Input: part model. Units: mm. Frame: model coordinates. A direction names the side the tool comes from. Coordinates: 2 decimals unless noted, no trailing zeros. Write each loop counter-clockwise with the first axis right and the second up, starting at its lowest first coordinate (ties: lowest second). Pieces come first, ordered by that corner, then holes. Notation, with made-up numbers: M -40,70.5 L -11,70.5 A25 cw -11,99.5 Z; hole C -30,-18.75 d6. An arc over 180 degrees is marked long. Answer as a JSON object with one key per item and string values. Group by question number.
from build123d import *

# Parameters (mm, degrees)
F0_W      = 20
F0_H      = 20
F0_R      = 3.5
F1_DEPTH  = 20
F2_R      = 3.5
F3_DEPTH  = 20
F4_R      = 3.5
F5_DEPTH  = 20
F6_R      = 5.5
F6_R_2    = 3.5
F7_DEPTH  = 16.5
F8_R      = 5.5
F9_DEPTH  = 16.5
F10_R     = 5.5
F11_DEPTH = 16.5


with BuildPart() as f1:
    # F0 (on Top) → F1 (new body)
    with BuildSketch(Plane.XY):
        Rectangle(F0_W, F0_H)
        Circle(F0_R, mode=Mode.SUBTRACT)
    extrude(amount=F1_DEPTH)

    # F2 (on face) → F3 (cut)
    with BuildSketch(Plane.XZ.offset(10)):
        with Locations((0, 10)):
            Circle(F2_R)
    extrude(amount=-F3_DEPTH, mode=Mode.SUBTRACT)

    # F4 (on face) → F5 (cut)
    with BuildSketch(Plane(origin=(-10, 0, 0), x_dir=(0, -1, 0), z_dir=(-1, 0, 0))):
        with Locations((0, 10)):
            Circle(F4_R)
    extrude(amount=-F5_DEPTH, mode=Mode.SUBTRACT)

    # F6 (on face) → F7 (cut)
    with BuildSketch(Plane.XY.offset(20)):
        Circle(F6_R)
        Circle(F6_R_2, mode=Mode.SUBTRACT)
    extrude(amount=-F7_DEPTH, mode=Mode.SUBTRACT)

    # F8 (on face) → F9 (cut)
    with BuildSketch(Plane(origin=(0, 10, 0), x_dir=(-1, 0, 0), z_dir=(0, 1, 0))):
        with Locations((0, 10)):
            Circle(F8_R)
    extrude(amount=-F9_DEPTH, mode=Mode.SUBTRACT)

    # F10 (on face) → F11 (cut)
    with BuildSketch(Plane.YZ.offset(10)):
        with Locations((0, 10)):
            Circle(F10_R)
    extrude(amount=-F11_DEPTH, mode=Mode.SUBTRACT)


solid = f1.part
Q1. Line query: line 1 (Z direction, x = 0, y = 8.5); line 2 (Y direction, x = 0, z = 16); line 3 (X direction, y = -3.75, z = 12). Output: solid intervals per line, ascending. Write a range as from..to.
Q2. Access query for faces 1 (the flat face through (-6.5, 4, 10)), 2 (the cylindrical face through (-4.05, 3.72, 17.67)), 3 (the cylindrical face through (4.05, 7.67, 13.72)). Directions: +Z, -Z, +X, -X, +Y, -Y. A direction counts if a zero-diameter tool reaches every point of the face in a straight line with its end or side. Return the directions, or none.
Q3. Pin query (flat end, axial travel): pin 1 Ø1 at (x, z) = (2, 12.5) entering from +Y; pin 2 Ø10 at (y, z) = (0, 10) entering from +X; pin 3 Ø9 at (x, y) = (1, 1) entering from +Z; pin 4 Ø10 at (x, y) = (0, 0) entering from +Z. Return the tip coordinate at first contact, or that it passes through.
Q4. Section D-D, the plane z = 1.5. Return the cut outline in (x, y), and give its area (3 significant figures).
Q5. Draft query along Y for faces 4 (the flat face through (-10, 0, 5)), 5 (the flat face through (-4, -6.5, 10)), 6 (the cylindrical face through (-5.495, 0.242, 4.244)). Return one class per face: released by +Y, released by -Y, zero draft, split by the parting line, or undercut.
Q6. Section B-B, the plane x = 0. Return the cut outline in (y, z).
Q7. Section A-A, the plane z = 10. Return the cut outline in (x, y), and give its area (3 significant figures).
Q8. Section C-C, the plane y = -8.5. Return the cut outline in (x, z), and give its area (3 significant figures).
Filled in:
{
 "1": {"line 1": "0..4.5, 15.5..20", "line 2": "-10..-5.5, 5.5..10", "line 3": "-10..-6.5"},
 "2": {"face 1": "+X", "face 2": "+Z", "face 3": "+Y"},
 "3": {"pin 1": "y = -6.5", "pin 2": "x = -6.5", "pin 3": "z = 20", "pin 4": "z = 3.5"},
 "4": {"outline": "M -10,-10 L 10,-10 L 10,10 L -10,10 Z; hole C 0,0 d7", "area": "362 mm^2"},
 "5": {"face 4": "zero draft", "face 5": "released by +Y", "face 6": "undercut"},
 "6": {"outline": "M -10,0 L -3.5,0 L -3.5,3.5 L -5.5,3.5 L -5.5,4.5 L -6.5,4.5 L -6.5,6.5 L -10,6.5 Z; M -10,13.5 L -6.5,13.5 L -6.5,15.5 L -5.5,15.5 L -5.5,20 L -10,20 Z; M 3.5,0 L 10,0 L 10,4.5 L 5.5,4.5 L 5.5,3.5 L 3.5,3.5 Z; M 5.5,15.5 L 10,15.5 L 10,20 L 5.5,20 Z"},
 "7": {"outline": "M -10,-10 L -3.5,-10 L -3.5,-6.5 L -5.5,-6.5 L -5.5,-5.5 L -6.5,-5.5 L -6.5,-3.5 L -10,-3.5 Z; M -10,3.5 L -6.5,3.5 L -6.5,5.5 L -5.5,5.5 L -5.5,10 L -10,10 Z; M 3.5,-10 L 10,-10 L 10,-5.5 L 5.5,-5.5 L 5.5,-6.5 L 3.5,-6.5 Z; M 5.5,5.5 L 10,5.5 L 10,10 L 5.5,10 Z", "area": "109 mm^2"},
 "8": {"outline": "M -10,0 L 10,0 L 10,20 L -10,20 Z; hole C 0,10 d7", "area": "362 mm^2"}
}
